```python
from build123d import *

# Parameters (mm, degrees)
F1_DEPTH = 135
F2_START = 25
F2_DEPTH = 110
F0_R     = 13.5
F3_DEPTH = 25
F4_W     = 20
F4_H     = 36.2463506984
F5_DEPTH = 2
F7_D     = 3
F7_DEPTH = 5
F7_TIP   = 0.9012909285
F9_D     = 10
F9_DEPTH = 20.001
F10_R    = 3


with BuildPart() as f1:
    # F0 (on Front) → F1 (new body)
    with BuildSketch(Plane.XZ):
        with BuildLine():
            ThreePointArc((-10, 17.3205080757), (-10, -17.3205080757), (20, 0))
            ThreePointArc((20, 0), (17.3205080757, 10), (10, 17.3205080757))
            Line((10, 17.3205080757), (10, 15.3205080757))
            Line((10, 15.3205080757), (9.448916991, 15.3205080757))
            ThreePointArc((9.448916991, 15.3205080757), (15.7175142093, 8.7726704646), (18, 0))
            ThreePointArc((18, 0), (-8.7726704646, -15.7175142093), (-9.448916991, 15.3205080757))
            Line((-9.448916991, 15.3205080757), (-10, 15.3205080757))
            Line((-10, 15.3205080757), (-10, 17.3205080757))
        make_face()
    extrude(amount=F1_DEPTH)

    # F0 (on Front) → F2 (join)
    with BuildSketch(Plane.XZ.offset(F2_START)):
        with BuildLine():
            Line((10, 15.3205080757), (10, 17.3205080757))
            ThreePointArc((10, 17.3205080757), (0, 20), (-10, 17.3205080757))
            Line((-10, 17.3205080757), (-10, 15.3205080757))
            Line((-10, 15.3205080757), (-9.448916991, 15.3205080757))
            ThreePointArc((-9.448916991, 15.3205080757), (0, 18), (9.448916991, 15.3205080757))
            Line((9.448916991, 15.3205080757), (10, 15.3205080757))
        make_face()
    extrude(amount=F2_DEPTH)

    # F0 (on Front) → F3 (join)
    with BuildSketch(Plane.XZ):
        with BuildLine():
            ThreePointArc((18, 0), (15.7175142093, 8.7726704646), (9.448916991, 15.3205080757))
            Line((9.448916991, 15.3205080757), (-9.448916991, 15.3205080757))
            ThreePointArc((-9.448916991, 15.3205080757), (-8.7726704646, -15.7175142093), (18, 0))
        make_face()
        Circle(F0_R, mode=Mode.SUBTRACT)
        Circle(F0_R)
    extrude(amount=F3_DEPTH)

    # F4 (on Front) → F5 (cut)
    with BuildSketch(Plane.XZ):
        with Locations((0, 3.1231753492)):
            Rectangle(F4_W, F4_H)
    extrude(amount=F5_DEPTH, mode=Mode.SUBTRACT)

    # F7
    with Locations(Plane.XY.offset(15.3205080757)):
        with Locations((4.2426406871, -10.7573593129), (-4.2426406871, -10.7573593129), (-4.2426406871, -19.2426406871), (4.2426406871, -19.2426406871)):
            Hole(F7_D / 2, depth=F7_DEPTH)
            with Locations((0, 0, -(F7_DEPTH + F7_TIP / 2))):  # 118° drill point
                Cone(0, F7_D / 2, F7_TIP, mode=Mode.SUBTRACT)

    # F9 (through all, one way)
    with BuildSketch(Plane(origin=(0, 0, 0), x_dir=(1, 0, 0), z_dir=(0, 0, -1))):
        with Locations((0, 35)):
            Circle(F9_D / 2)
    extrude(amount=-F9_DEPTH, mode=Mode.SUBTRACT)

    # F10
    f10_edges = [f1.edges().sort_by_distance(p)[0] for p in [
        (0, -2, 15.320508),
    ]]
    fillet(f10_edges, radius=F10_R)


solid = f1.part
```
Part model, mm, in its own coordinate system. A direction names the side the tool comes from. Round coordinates to 2 decimals unless told otherwise and drop trailing zeros. Write each loop counter-clockwise with the first axis right and the second up, starting at its lowest first coordinate (ties: lowest second). Pieces come first, ordered by that corner, then holes. Notation, with made-up numbers: M 47.5,55 L 55.5,55 A10 cw 55.5,59 Z; hole C -15,-11 d5. An arc over 180 degrees is marked long. One line per question, with ' | ' between items.
(1) Saw through at A-A on x = 0. Write the cut outline in (y, z), then the cut area to 3 significant figures.
Answer key:
outline: M -135,-20 L 0,-20 L 0,-15 L -2,-15 L -2,12.32 A3 ccw -5,15.32 L -25,15.32 L -25,-18 L -135,-18 Z; M -135,18 L -40,18 L -40,20 L -135,20 Z; M -30,18 L -25,18 L -25,20 L -30,20 Z | area: 1,240 mm^2
(2) Probe line 1 along Z through (x, y) = (-1, -77); line 2 along Y through (x, z) = (-6.5, 7.5). List the from-to ranges inside material, lowest first.
Answer key:
line 1: z = -19.97 to -17.97, 17.97 to 19.97 | line 2: y = -25 to -2
(3) Saw through at B-B on z = -7. Write the cut outline in (x, y) (3 decimals).
Answer key:
outline: M -18.735,-135 L -16.583,-135 L -16.583,-25 L 16.583,-25 L 16.583,-135 L 18.735,-135 L 18.735,0 L 10,0 L 10,-2 L -10,-2 L -10,0 L -18.735,0 Z
(4) Two-plate mould, pull along X, no slides. Class faces 1 (the face through (-4.1, -19.02, 9.58)), 2 (the face through (10.3, 0, -4)): released by +X, released by -X, zero draft, split by the parting line, or undercut.
Answer key:
face 1: undercut | face 2: zero draft
(5) 3-axis set-ups, long thin cutter, end or side, ignore diameter. For faces 3 (the face through (0, -25, -1)), 4 (the face through (-4.047, -17.755, 12.786)), 5 (the face through (10, -1, 8)): which of +Z, -Z, +X, -X, +Y, -Y reach the whole face in a straight line?
Answer key:
face 3: -Y | face 4: +Z | face 5: +Z, +Y
(6) Saw through at C-C on y = -35. Write the cut outline in (x, z).
Answer key:
outline: M -5,17.29 L -5,19.36 A20 ccw long 5,19.36 L 5,17.29 A18 cw long Z
(7) Saw through at D-D on x = 7.5. Write the cut outline in (y, z).
Answer key:
outline: M -135,-18.54 L 0,-18.54 L 0,-15 L -2,-15 L -2,12.32 A3 ccw -5,15.32 L -25,15.32 L -25,-16.36 L -135,-16.36 Z; M -135,16.36 L -25,16.36 L -25,18.54 L -135,18.54 Z
(8) Pin check, flat tips, straight feed: pin 1 (5 mm diameter, centred on x = -1.5, z = 16.5, fed in from +Y); pin 2 (3 mm diameter, centred on x = -4, z = -5.5, fed in from +Y); pin 3 (10 mm diameter, centred on x = -11.5, y = -21.5, fed in from -Z); pin 4 (10 mm diameter, centred on y = -103.5, z = 1.5, fed in from +X). Stop position of each tip, or through.
Answer key:
pin 1: stops at y = -2.51 | pin 2: stops at y = -2 | pin 3: stops at z = -18.91 | pin 4: stops at x = 20
